Could you check a few things on this drawing? It's one solid part, dimensions in mm from its lowest x, y, z. A direction names the side the tool comes from. Coordinates: 2 decimals unless noted, no trailing zeros. Order: outer loops, then holes, each group sorted by start corner. A loop starts at its lowest first (then second) coordinate and runs counter-clockwise, first axis right, second up. Notation, with made-up numbers: (86, 10) - (108, 10) arc R32 cw to (108, 47) - close; hole circle Ø4 at (20, 8.25). An arc over 180 degrees is marked (long way). Return JSON: item names as keys, results as strings. Group by question number.
1) For pin 1 Ø4 at (y, z) = (4, 9.5) entering from -X; pin 2 Ø5 at (x, z) = (5, 9) entering from +Y; pin 3 Ø0.6 at (x, z) = (33.5, 10.5) entering from +Y; pin 4 Ø1 at (y, z) = (3, 5.5) entering from -X, each with a flat end and sliding along its axis, tell me the tip position at first contact or that it passes through.
2) If I drill on line 1 along Y through (x, z) = (9, 13.5); line 2 along X through (y, z) = (5.5, 4); line 3 along X through (y, z) = (3, 12), over which ranges is the centre line in solid material (lowest first)?
3) Which directions (+Z, -Z, +X, -X, +Y, -Y) give clear straight access to the entire face, cutting with the end or side of a thin tool? Please do the marked faces 1 and 2.
4) Imagine slicing it at B-B (x = 3). Write out the boundary of the cut face in (y, z), and give its area (3 significant figures).
5) Imagine slicing it at D-D (x = 27). Write out the boundary of the cut face in (y, z), and give its area (3 significant figures).
6) Imagine slicing it at A-A (y = 5.25). Write out the boundary of the cut face in (x, z).
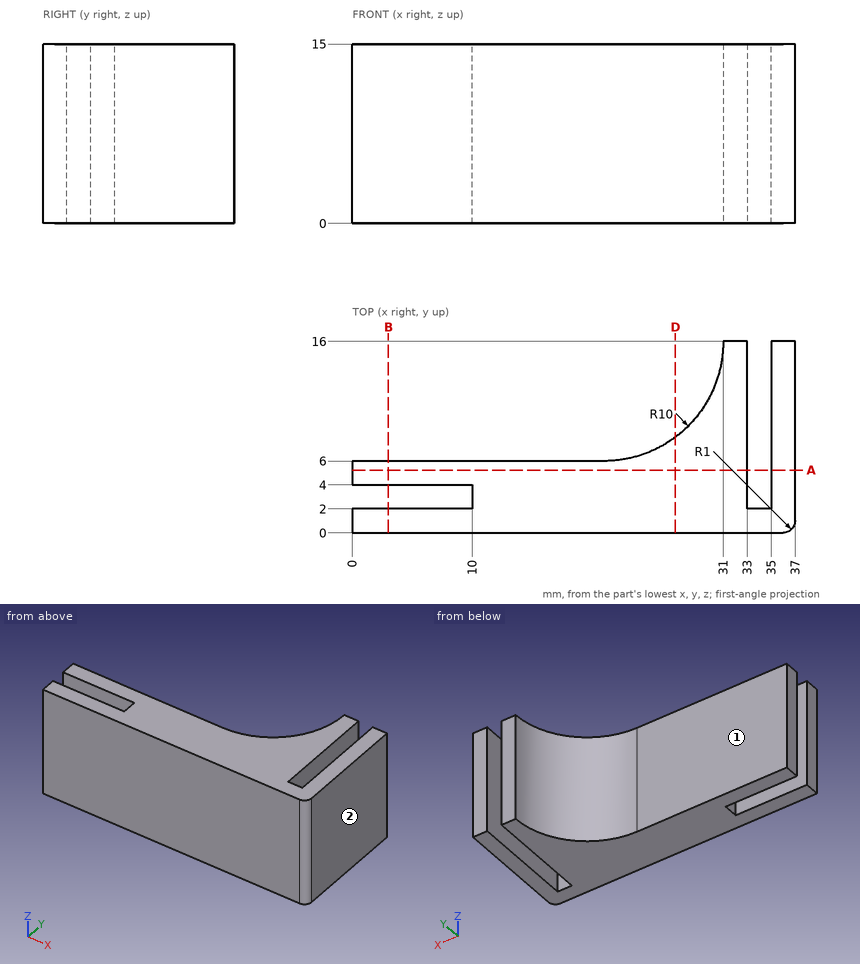
Calculated:
{
 "1": {"pin 1": "x = 0", "pin 2": "y = 6", "pin 3": "y = 2", "pin 4": "x = 10"},
 "2": {"line 1": "0 to 2, 4 to 6", "line 2": "0 to 33, 35 to 37", "line 3": "10 to 33, 35 to 37"},
 "3": {"face 1": "+Z, -Z, -X, +Y", "face 2": "+Z, -Z, +X, +Y, -Y"},
 "4": {"outline": "(0, 0) - (2, 0) - (2, 15) - (0, 15) - close; (4, 0) - (6, 0) - (6, 15) - (4, 15) - close", "area": "60.0 mm2"},
 "5": {"outline": "(0, 0) - (8, 0) - (8, 15) - (0, 15) - close", "area": "120 mm2"},
 "6": {"outline": "(0, 0) - (33, 0) - (33, 15) - (0, 15) - close; (35, 0) - (37, 0) - (37, 15) - (35, 15) - close"}
}
